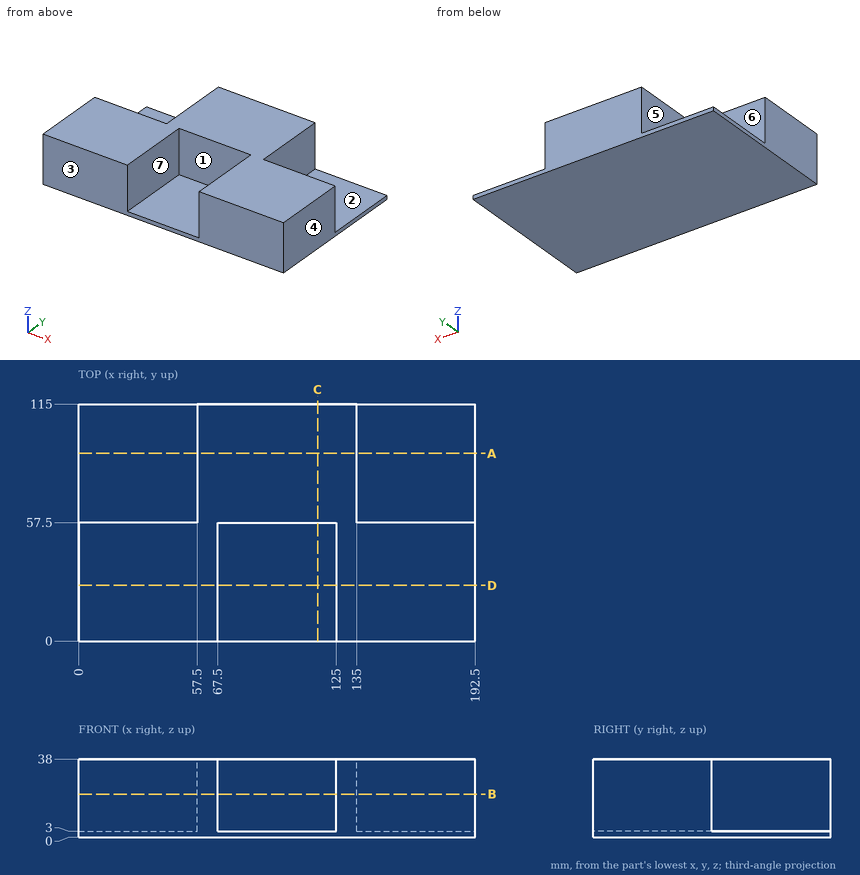
The drawing under review shows one solid part. Ordinate dimensions are in mm from its lowest x, y, z. A direction names the side the tool comes from. Give positions to 0.01 mm unless a question says otherwise; leave off trailing zeros. Order: outer loops, then holes, each group sorted by start corner. A loop starts at its lowest first (then second) coordinate and runs counter-clockwise, first axis right, second up. Notation, with made-up numbers: (-23, 13.5) - (22, 13.5) arc R12 ccw to (22, 27.5) - close; hole circle Ø1 at (20.5, 73). An arc over 180 degrees is marked (long way). Answer as a JSON object with one key per item and string values. Group by question number.
Item 1: Draft analysis for pull direction X (two halves, no side actions). For the marked faces 4, 5, 6 and 7, state which applies: pulls with the +X half, pulls with the -X half, needs draft (parallel to the pull), parting line crosses it, or undercut.
Item 2: Take a section at D-D on y = 27. Give the boundary of the cut face in (x, z), and give its area (3 significant figures).
Item 3: Take a section at C-C on x = 116. Give the boundary of the cut face in (y, z), and give its area (3 significant figures).
Item 4: Wall thickness on line 1 along X through (y, z) = (41, 5.5); line 2 along X through (y, z) = (81, 35); line 3 along Y through (x, z) = (121, 33): over which ranges is each line inside the solid? List them lowest first.
Item 5: Clearance check with flat-ended pins moving along their axes: pin 1 Ø12 at (y, z) = (16.5, 9.5) entering from -X; pin 2 Ø17.5 at (x, z) = (177, 17.5) entering from +Y; pin 3 Ø10.5 at (x, z) = (96, 25) entering from -Y; pin 4 Ø1.5 at (y, z) = (80.5, 22) entering from +X. State where each tip first meets the part, or that it passes through.
Item 6: Take a section at B-B on z = 21. Give the boundary of the cut face in (x, y), and give its area (3 significant figures).
Item 7: Take a section at A-A on y = 91. Give the boundary of the cut face in (x, z).
Item 8: Machinability: for the marked faces 1, 2 and 3, which of the approach directions +Z, -Z, +X, -X, +Y, -Y give a long, thin tool a straight path to every point of the face, cutting with its end or side? Answer none if there is none.
Reported:
{
 "1": {"face 4": "pulls with the +X half", "face 5": "pulls with the -X half", "face 6": "needs draft", "face 7": "undercut"},
 "2": {"outline": "(0, 0) - (192.5, 0) - (192.5, 38) - (125, 38) - (125, 3) - (67.5, 3) - (67.5, 38) - (0, 38) - close", "area": "5,300 mm^2"},
 "3": {"outline": "(0, 0) - (115, 0) - (115, 38) - (57.5, 38) - (57.5, 3) - (0, 3) - close", "area": "2,360 mm^2"},
 "4": {"line 1": "0 to 67.5, 125 to 192.5", "line 2": "57.5 to 135", "line 3": "57.5 to 115"},
 "5": {"pin 1": "x = 0", "pin 2": "y = 57.5", "pin 3": "y = 57.5", "pin 4": "x = 135"},
 "6": {"outline": "(0, 0) - (67.5, 0) - (67.5, 57.5) - (125, 57.5) - (125, 0) - (192.5, 0) - (192.5, 57.5) - (135, 57.5) - (135, 115) - (57.5, 115) - (57.5, 57.5) - (0, 57.5) - close", "area": "12,200 mm^2"},
 "7": {"outline": "(0, 0) - (192.5, 0) - (192.5, 3) - (135, 3) - (135, 38) - (57.5, 38) - (57.5, 3) - (0, 3) - close"},
 "8": {"face 1": "+Z, -Y", "face 2": "+Z, +X, +Y", "face 3": "+Z, -Z, +X, -X, -Y"}
}
